```python
from build123d import *

# Parameters (mm, degrees)
SKETCH1_W           = 152
SKETCH1_H           = 132
SKETCH1_W_2         = 150
SKETCH1_H_2         = 130
BOSS_EXTRUDE1_DEPTH = 3
SKETCH2_W           = 152
SKETCH2_H           = 132
SKETCH2_W_2         = 141
SKETCH2_H_2         = 121
BOSS_EXTRUDE2_DEPTH = 1
FILLET1_R           = 1.4
FILLET2_R           = 3


with BuildPart() as part:
    # Sketch1 → Boss-Extrude1 (new body)
    with BuildSketch(Plane.XY):
        with Locations((-0.37936772, -7.96672213)):
            Rectangle(SKETCH1_W, SKETCH1_H)
        with Locations((-0.37936772, -7.96672213)):
            Rectangle(SKETCH1_W_2, SKETCH1_H_2, mode=Mode.SUBTRACT)
    extrude(amount=BOSS_EXTRUDE1_DEPTH)

    # Sketch2 → Boss-Extrude2 (add)
    with BuildSketch(Plane.XY.offset(3)):
        with Locations((-0.37936772, -7.96672213)):
            Rectangle(SKETCH2_W, SKETCH2_H)
        with Locations((-0.37936772, -7.96672213)):
            Rectangle(SKETCH2_W_2, SKETCH2_H_2, mode=Mode.SUBTRACT)
    extrude(amount=BOSS_EXTRUDE2_DEPTH)

    # Fillet1
    fillet1_edges = [part.edges().sort_by_distance(p)[0] for p in [
        (-75.37936772, 57.03327787, 1.5),
        (-75.37936772, -72.96672213, 1.5),
        (74.62063228, -72.96672213, 1.5),
        (74.62063228, 57.03327787, 1.5),
        (-75.37936772, -7.96672213, 3),
        (-0.37936772, -72.96672213, 3),
        (74.62063228, -7.96672213, 3),
        (-0.37936772, 57.03327787, 3),
    ]]
    fillet(fillet1_edges, radius=FILLET1_R)

    # Fillet2
    fillet2_edges = [part.edges().sort_by_distance(p)[0] for p in [
        (-76.37936772, -7.96672213, 4),
        (-0.37936772, -73.96672213, 4),
        (75.62063228, -7.96672213, 4),
        (-0.37936772, 58.03327787, 4),
        (-76.37936772, 58.03327787, 2),
        (75.62063228, 58.03327787, 2),
        (75.62063228, -73.96672213, 2),
        (-76.37936772, -73.96672213, 2),
    ]]
    fillet(fillet2_edges, radius=FILLET2_R)


solid = part.part
```
Can you work these out from the model? Positions are in its coordinate system, mm. Round coordinates to 2 decimals unless told otherwise and drop trailing zeros. Order: outer loops, then holes, each group sorted by start corner. A loop starts at its lowest first (then second) coordinate and runs counter-clockwise, first axis right, second up. Notation, with made-up numbers: (7, 4.5) -> (57, 4.5) arc R24 ccw to (57, 37.5) -> close; hole circle Ø7 at (4, 73). An arc over 180 degrees is marked (long way). Return JSON: item names as keys, results as strings. Group by question number.
1. I need wall thicknesses on line 1 (X direction, y = 1, z = 3.25); line 2 (Y direction, x = -4, z = 0.55); line 3 (Y direction, x = 24, z = 1.45). Which ranges of each line are inside material? Lowest first, please. Write a range as [from, to].
2. We'd pull the mould along X, two halves only. Please class faces 1 (the face through (-6, -69, 3)), 2 (the face through (-33, 53, 4)): released by +X, released by -X, zero draft, split by the parting line, or undercut.
3. If we section it at A-A, the plane x = 45.5: Write out the boundary of the cut face in (y, z).
4. Will these pins go through, and if not, where does the flat tip stop? pin 1 (1 mm diameter, centred on y = 42, z = 3, fed in from -X); pin 2 (1.1 mm diameter, centred on x = 34.5, z = 3.5, fed in from +Y); pin 3 (1.1 mm diameter, centred on y = -36, z = 3.5, fed in from +X).
5. If we section it at B-B, the plane y = -16.5: Write out the boundary of the cut face in (x, z), then the cut area to 3 significant figures.
Output values:
{
 "1": {"line 1": "[-75.36, -70.88], [70.12, 74.6]", "line 2": "[-73.97, -72.97], [57.03, 58.03]", "line 3": "[-73.93, -72.97], [57.03, 58]"},
 "2": {"face 1": "undercut", "face 2": "zero draft"},
 "3": {"outline": "(-73.97, 0) -> (-72.97, 0) -> (-72.97, 1.6) arc R1.4 cw to (-71.57, 3) -> (-68.47, 3) -> (-68.47, 4) -> (-70.97, 4) arc R3 ccw to (-73.97, 1) -> close; (52.53, 3) -> (55.63, 3) arc R1.4 cw to (57.03, 1.6) -> (57.03, 0) -> (58.03, 0) -> (58.03, 1) arc R3 ccw to (55.03, 4) -> (52.53, 4) -> close"},
 "4": {"pin 1": "x = -75.98", "pin 2": "y = 57.31", "pin 3": "x = 74.9"},
 "5": {"outline": "(-76.38, 0) -> (-75.38, 0) -> (-75.38, 1.6) arc R1.4 cw to (-73.98, 3) -> (-70.88, 3) -> (-70.88, 4) -> (-73.38, 4) arc R3 ccw to (-76.38, 1) -> close; (70.12, 3) -> (73.22, 3) arc R1.4 cw to (74.62, 1.6) -> (74.62, 0) -> (75.62, 0) -> (75.62, 1) arc R3 ccw to (72.62, 4) -> (70.12, 4) -> close", "area": "14.0 mm²"}
}
